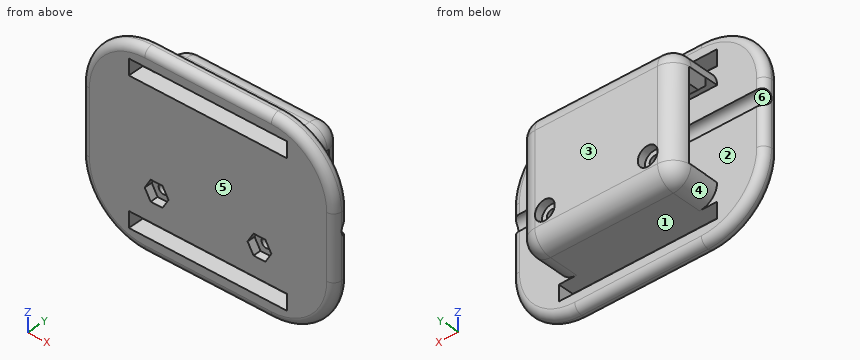
from build123d import *

# Parameters (mm, degrees)
SKETCH1_W               = 31.75
SKETCH1_H               = 25.4
BOSS_EXTRUDE1_DEPTH     = 12.7
SKETCH2_W               = 18.25625
SKETCH2_H               = 6.35
CUT_EXTRUDE3_DEPTH      = 39.058949894
SKETCH4_W               = 1.5875
SKETCH4_H               = 4.7625
BOSS_EXTRUDE2_DEPTH     = 31.75
CUT_EXTRUDE5_DEPTH      = 31.590858593
CUT_EXTRUDE5_DEPTH_BACK = 31.590858593
SKETCH5_R               = 0.9921875
CUT_EXTRUDE6_DEPTH      = 1.5875
SKETCH7_R               = 1.984375
CUT_EXTRUDE7_DEPTH      = 1.5875
SKETCH8_W               = 50.8
SKETCH8_H               = 38.305926372
SKETCH8_W_2             = 31.75
SKETCH8_H_2             = 25.4
BOSS_EXTRUDE3_DEPTH     = 3.175
SKETCH10_W              = 31.75
SKETCH10_H              = 3.175
CUT_EXTRUDE8_DEPTH      = 42.677098196
FILLET6_R               = 12.7
CHAMFER1_SIZE           = 1.016
CHAMFER2_SIZE           = 1.524
FILLET7_R               = 3.556
FILLET10_R              = 1.5875
SKETCH13_R              = 1.5875
CUT_EXTRUDE9_DEPTH      = 74.216005252


# Some blends are built 0.0001 mm under size
with BuildPart() as part:
    # Sketch1 → Boss-Extrude1 (new body)
    with BuildSketch(Plane(origin=(0, 0, 0), x_dir=(1, 0, 0), z_dir=(0, 1, 0))):
        with Locations((7.914574134, 4.007219009)):
            Rectangle(SKETCH1_W, SKETCH1_H)
    extrude(amount=BOSS_EXTRUDE1_DEPTH)

    # Sketch2 → Cut-Extrude3 (cut, through all)
    with BuildSketch(Plane(origin=(23.789574134, 0, 0), x_dir=(0, 0, -1), z_dir=(1, 0, 0))):
        with Locations((4.007219009, 6.35)):
            Rectangle(SKETCH2_W, SKETCH2_H)
    extrude(amount=-CUT_EXTRUDE3_DEPTH, mode=Mode.SUBTRACT)

    # Sketch4 → Boss-Extrude2 (add, through all)
    with BuildSketch(Plane(origin=(23.789574134, 0, 0), x_dir=(0, 0, -1), z_dir=(1, 0, 0))):
        with Locations((-4.327155991, 7.14375)):
            Rectangle(SKETCH4_W, SKETCH4_H)
        with Locations((12.341594009, 7.14375)):
            Rectangle(SKETCH4_W, SKETCH4_H)
    extrude(amount=-BOSS_EXTRUDE2_DEPTH)

    # Sketch5 → Cut-Extrude5 (cut, two sides: drawn at the far end of the back side and taken through both)
    with BuildSketch(Plane(origin=(0, 3.175, 0), x_dir=(1, 0, 0), z_dir=(0, 1, 0)).offset(-CUT_EXTRUDE5_DEPTH_BACK)):
        with Locations(Location((-2.404175866, 10.754094009, 0), (0, 0, 270))):
            Circle(SKETCH5_R)
        with Locations(Location((18.233324134, 10.754094009, 0), (0, 0, 126.869897646))):
            Circle(SKETCH5_R)
    extrude(amount=CUT_EXTRUDE5_DEPTH + CUT_EXTRUDE5_DEPTH_BACK, mode=Mode.SUBTRACT)

    # Sketch6 → Cut-Extrude6 (cut)
    with BuildSketch(Plane.XZ):
        Polygon((-0.022925866, -10.754094009), (-1.213550866, -8.691871016), (-3.594800866, -8.691871016), (-4.785425866, -10.754094009), (-3.594800866, -12.816317002), (-1.213550866, -12.816317002), align=None)
        Polygon((20.614574134, -10.754094009), (19.423949134, -8.691871016), (17.042699134, -8.691871016), (15.852074134, -10.754094009), (17.042699134, -12.816317002), (19.423949134, -12.816317002), align=None)
    extrude(amount=-CUT_EXTRUDE6_DEPTH, mode=Mode.SUBTRACT)

    # Sketch7 → Cut-Extrude7 (cut)
    with BuildSketch(Plane(origin=(0, 12.7, 0), x_dir=(1, 0, 0), z_dir=(0, 1, 0))):
        with Locations(Location((-2.404175866, 10.754094009, 0), (0, 0, 270))):
            Circle(SKETCH7_R)
        with Locations(Location((18.233324134, 10.754094009, 0), (0, 0, 270))):
            Circle(SKETCH7_R)
    extrude(amount=-CUT_EXTRUDE7_DEPTH, mode=Mode.SUBTRACT)

    # Sketch8 → Boss-Extrude3 (add)
    with BuildSketch(Plane.XZ):
        with Locations((7.914574134, -4.007219009)):
            Rectangle(SKETCH8_W, SKETCH8_H)
        with Locations((7.914574134, -4.007219009)):
            Rectangle(SKETCH8_W_2, SKETCH8_H_2, mode=Mode.SUBTRACT)
    extrude(amount=-BOSS_EXTRUDE3_DEPTH)

    # Sketch10 → Cut-Extrude8 (cut, through all)
    with BuildSketch(Plane(origin=(0, 3.175, 0), x_dir=(1, 0, 0), z_dir=(0, 1, 0))):
        with Locations((7.914574134, 18.294719009)):
            Rectangle(SKETCH10_W, SKETCH10_H)
        with Locations((7.914574134, -10.280280991)):
            Rectangle(SKETCH10_W, SKETCH10_H)
    extrude(amount=-CUT_EXTRUDE8_DEPTH, mode=Mode.SUBTRACT)

    # Fillet6
    fillet6_edges = [part.edges().sort_by_distance(p)[0] for p in [
        (-17.485425866, 1.5875, 15.145744177),
        (33.314574134, 1.5875, 15.145744177),
        (33.314574134, 1.5875, -23.160182195),
        (-17.485425866, 1.5875, -23.160182195),
    ]]
    fillet(fillet6_edges, radius=FILLET6_R)

    # Chamfer1
    # the kernel refuses this chamfer: 1.016 mm, written as the material it takes off along each edge
    with BuildSketch(Plane(origin=(-7.960425866, 4.7625, 0.920576075), x_dir=(-0.027495876610586435, 0.9996219169112968, 0), z_dir=(0, 0, 1)), Plane(origin=(-7.960425866, 4.7625, -13.135344009), x_dir=(-0.027495876610586435, 0.9996219169112968, 1.1185418764848949e-15), z_dir=(0, 0, 1))) as chamfer1_piece_1:
        Polygon((CHAMFER1_SIZE * 0.999621916911, -CHAMFER1_SIZE * 0.0274958766106), (-CHAMFER1_SIZE * 0.0274958766106, -CHAMFER1_SIZE * 0.999621916911), (0, 0), align=None)
    extrude(amount=4.200329916, mode=Mode.SUBTRACT)
    with BuildSketch(Plane(origin=(26.402404049, 4.7625, 3.533405991), x_dir=(0, 0.9996219169112968, -0.027495876610586435), z_dir=(-1, 0, 0))) as chamfer1_piece_2:
        Polygon((CHAMFER1_SIZE * 0.999621916911, -CHAMFER1_SIZE * 0.0274958766106), (-CHAMFER1_SIZE * 0.0274958766106, -CHAMFER1_SIZE * 0.999621916911), (0, 0), align=None)
    extrude(amount=36.975659832, mode=Mode.SUBTRACT)
    with BuildSketch(Plane(origin=(23.789574134, 4.7625, 0.920576075), x_dir=(0.027495876610587285, 0.9996219169112968, 0), z_dir=(0, 0, 1)), Plane(origin=(23.789574134, 4.7625, -13.135344009), x_dir=(0.027495876610587285, 0.9996219169112968, 1.1185418764848949e-15), z_dir=(0, 0, 1))) as chamfer1_piece_3:
        Polygon((CHAMFER1_SIZE * 0.999621916911, CHAMFER1_SIZE * 0.0274958766106), (-CHAMFER1_SIZE * 0.0274958766106, CHAMFER1_SIZE * 0.999621916911), (0, 0), align=None)
    extrude(amount=4.200329916, mode=Mode.SUBTRACT)
    with BuildSketch(Plane(origin=(-0.386658451, 4.7625, -11.547844009), x_dir=(0, -0.027495876610585605, -0.9996219169112968), z_dir=(-1, 0, 0)), Plane(origin=(26.402404049, 4.7625, -11.547844009), x_dir=(0, -0.027495876610585605, -0.9996219169112968), z_dir=(-1, 0, 0))) as chamfer1_piece_4:
        Polygon((CHAMFER1_SIZE * 0.999621916911, -CHAMFER1_SIZE * 0.0274958766106), (-CHAMFER1_SIZE * 0.0274958766106, -CHAMFER1_SIZE * 0.999621916911), (0, 0), align=None)
    extrude(amount=10.186597332, mode=Mode.SUBTRACT)
    with BuildSketch(Plane(origin=(20.250841549, 4.7625, -11.547844009), x_dir=(0, -0.027495876610585605, -0.9996219169112968), z_dir=(-1, 0, 0))) as chamfer1_piece_5:
        Polygon((CHAMFER1_SIZE * 0.999621916911, -CHAMFER1_SIZE * 0.0274958766106), (-CHAMFER1_SIZE * 0.0274958766106, -CHAMFER1_SIZE * 0.999621916911), (0, 0), align=None)
    extrude(amount=24.672534832, mode=Mode.SUBTRACT)

    # Chamfer2
    chamfer2_edges = [part.edges().sort_by_distance(p)[0] for p in [
        (-7.960425866, 7.65175, 3.533405991),
        (23.789574134, 7.65175, 3.533405991),
        (-7.960425866, 7.65175, -11.547844009),
        (23.789574134, 7.65175, -11.547844009),
    ]]
    chamfer(chamfer2_edges, length=CHAMFER2_SIZE)

    # Fillet7
    # the kernel refuses this fillet: 3.556 mm, written as the material it takes off along each edge
    with BuildSketch(Plane(origin=(20.233574134, 9.144, 5.136780991), x_dir=(0, 0, 1), z_dir=(1, 0, 0))) as fillet7_piece_1_section:
        Polygon((0, 0), (FILLET7_R * 1.02, 0), (FILLET7_R * 1.02, -FILLET7_R * 1.02), (0, -FILLET7_R * 1.02), align=None)
    fillet7_piece_1 = extrude(amount=FILLET7_R * 1.02, mode=Mode.PRIVATE)
    fillet7_piece_1 = fillet7_piece_1 - Plane(origin=(20.233574134, 9.144, 5.136780991), x_dir=(0, -0.7071067811865475, -0.7071067811865475), z_dir=(1, 0, 0)) * Sphere(FILLET7_R, mode=Mode.PRIVATE)
    add(fillet7_piece_1, mode=Mode.SUBTRACT)
    with BuildSketch(Plane(origin=(-4.404425866, 9.144, 5.136780991), x_dir=(0, 0, 1), z_dir=(-1, 0, 0))) as fillet7_piece_2_section:
        Polygon((0, 0), (FILLET7_R * 1.02, 0), (FILLET7_R * 1.02, FILLET7_R * 1.02), (0, FILLET7_R * 1.02), align=None)
    fillet7_piece_2 = extrude(amount=FILLET7_R * 1.02, mode=Mode.PRIVATE)
    fillet7_piece_2 = fillet7_piece_2 - Plane(origin=(-4.404425866, 9.144, 5.136780991), x_dir=(0, -0.7071067811865475, -0.7071067811865475), z_dir=(-1, 0, 0)) * Sphere(FILLET7_R, mode=Mode.PRIVATE)
    add(fillet7_piece_2, mode=Mode.SUBTRACT)
    with BuildSketch(Plane(origin=(20.233574134, 9.144, -13.151219009), x_dir=(1, 0, 0), z_dir=(0, 0, -1))) as fillet7_piece_3_section:
        Polygon((0, 0), (FILLET7_R * 1.02, 0), (FILLET7_R * 1.02, -FILLET7_R * 1.02), (0, -FILLET7_R * 1.02), align=None)
    fillet7_piece_3 = extrude(amount=FILLET7_R * 1.02, mode=Mode.PRIVATE)
    fillet7_piece_3 = fillet7_piece_3 - Plane(origin=(20.233574134, 9.144, -13.151219009), x_dir=(-0.7071067811865475, -0.7071067811865475, 0), z_dir=(0, 0, -1)) * Sphere(FILLET7_R, mode=Mode.PRIVATE)
    add(fillet7_piece_3, mode=Mode.SUBTRACT)
    with BuildSketch(Plane(origin=(-4.404425866, 9.144, -13.151219009), x_dir=(-1, 0, 0), z_dir=(0, 0, -1))) as fillet7_piece_4_section:
        Polygon((0, 0), (FILLET7_R * 1.02, 0), (FILLET7_R * 1.02, FILLET7_R * 1.02), (0, FILLET7_R * 1.02), align=None)
    fillet7_piece_4 = extrude(amount=FILLET7_R * 1.02, mode=Mode.PRIVATE)
    fillet7_piece_4 = fillet7_piece_4 - Plane(origin=(-4.404425866, 9.144, -13.151219009), x_dir=(0.7071067811865475, -0.7071067811865475, 0), z_dir=(0, 0, -1)) * Sphere(FILLET7_R, mode=Mode.PRIVATE)
    add(fillet7_piece_4, mode=Mode.SUBTRACT)
    with BuildSketch(Plane(origin=(20.233574134, 12.7, 8.692780991), x_dir=(0, -1, 0), z_dir=(-1, 0, 0))) as fillet7_piece_5:
        with BuildLine():
            CenterArc((FILLET7_R, -FILLET7_R), FILLET7_R, 90, 90)
            Line((0, -FILLET7_R), (0, 0))
            Line((0, 0), (FILLET7_R, 0))
        make_face()
    extrude(amount=24.638, mode=Mode.SUBTRACT)
    with BuildSketch(Plane(origin=(23.789574134, 3.175, 8.692780991), x_dir=(-1, 0, 0), z_dir=(0, 1, 0)), Plane(origin=(-7.960425866, 3.175, -16.707219009), x_dir=(1, 0, 0), z_dir=(0, 1, 0))) as fillet7_piece_6:
        with BuildLine():
            CenterArc((FILLET7_R, -FILLET7_R), FILLET7_R, 90, 90)
            Line((0, -FILLET7_R), (0, 0))
            Line((0, 0), (FILLET7_R, 0))
        make_face()
    extrude(amount=5.969, mode=Mode.SUBTRACT)
    with BuildSketch(Plane(origin=(23.789574134, 12.7, -13.151219009), x_dir=(-1, 0, 0), z_dir=(0, 0, 1)), Plane(origin=(-7.960425866, 12.7, 5.136780991), x_dir=(1, 0, 0), z_dir=(0, 0, -1))) as fillet7_piece_7:
        with BuildLine():
            CenterArc((FILLET7_R, FILLET7_R), FILLET7_R, 180, 90)
            Line((0, FILLET7_R), (0, 0))
            Line((0, 0), (FILLET7_R, 0))
        make_face()
    extrude(amount=18.288, mode=Mode.SUBTRACT)
    with BuildSketch(Plane(origin=(23.789574134, 3.175, -16.707219009), x_dir=(-1, 0, 0), z_dir=(0, 1, 0)), Plane(origin=(-7.960425866, 3.175, 8.692780991), x_dir=(1, 0, 0), z_dir=(0, 1, 0))) as fillet7_piece_8:
        with BuildLine():
            CenterArc((FILLET7_R, FILLET7_R), FILLET7_R, 180, 90)
            Line((0, FILLET7_R), (0, 0))
            Line((0, 0), (FILLET7_R, 0))
        make_face()
    extrude(amount=5.969, mode=Mode.SUBTRACT)
    with BuildSketch(Plane(origin=(-4.404425866, 12.7, -16.707219009), x_dir=(0, 0, 1), z_dir=(1, 0, 0))) as fillet7_piece_9:
        with BuildLine():
            CenterArc((FILLET7_R, FILLET7_R), FILLET7_R, 180, 90)
            Line((0, FILLET7_R), (0, 0))
            Line((0, 0), (FILLET7_R, 0))
        make_face()
    extrude(amount=24.638, mode=Mode.SUBTRACT)

    # Fillet10
    fillet10_edges = [part.edges().sort_by_distance(p)[0] for p in [
        (7.914574134, 3.175, 15.145744177),
        (7.914574134, 0, 15.145744177),
        (-17.485425866, 0, -4.007219009),
        (7.914574134, 0, -23.160182195),
        (33.314574134, 0, -4.007219009),
        (29.594830255, 0, 11.426000298),
        (29.594830255, 0, -19.440438316),
        (-13.765681988, 0, -19.440438316),
        (-13.765681988, 0, 11.426000298),
        (-17.485425866, 3.175, -4.007219009),
        (33.314574134, 3.175, -4.007219009),
        (7.914574134, 3.175, -23.160182195),
    ]]
    fillet(fillet10_edges, radius=FILLET10_R - 0.0001)  # a hair under: the kernel refuses the full size

    # Sketch13 → Cut-Extrude9 (cut, through all)
    with BuildSketch(Plane(origin=(50.8, 0, 0), x_dir=(0, 0, -1), z_dir=(1, 0, 0))):
        with Locations((1.213219009, 3.175)):
            Circle(SKETCH13_R)
    extrude(amount=-CUT_EXTRUDE9_DEPTH, mode=Mode.SUBTRACT)


solid = part.part
Could you check a few things on this model? Use its own coordinates, in mm. Face numbers are marked on the shaded views. A direction names the side the tool comes from. Coordinates: 2 decimals unless noted, no trailing zeros. Order: outer loops, then holes, each group sorted by start corner. A loop starts at its lowest first (then second) coordinate and runs counter-clockwise, first axis right, second up. Notation, with made-up numbers: (61.5, 21.25) -> (96.5, 21.25) arc R15 cw to (96.5, 38.25) -> close; hole circle Ø9 at (-39, 7.25). An arc over 180 degrees is marked (long way). One line per item, written item: value. Start each with the question number.
1) Imagine slicing it at B-B on y = 6.75. List the corners of the cut face in (x, z) for me, plus the area to 3 significant figures.
2) I'm going to push flat-ended pins straight in: pin 1 (4 mm diameter, centred on x = 6, y = 7.5, fed in from +Z); pin 2 (2.5 mm diameter, centred on x = 18.23, z = -10.75, fed in from +Y); pin 3 (3.5 mm diameter, centred on y = 1.5, z = 10.5, fed in from -X); pin 4 (1.2 mm diameter, centred on x = -2.4, z = -10.75, fed in from -Y). Where does each tip first touch, or does it pass through?
3) We'd pull the mould along Z, two halves only. Please class the marked faces 1, 2, 3 and 4: +Z half, -Z half, draft (parallel to the pull), parting line (faces both ways), or undercut.
4) Which directions (+Z, -Z, +X, -X, +Y, -Y) give clear straight access to the entire face, cutting with the end or side of a thin tool? Please do the marked faces 5 and 6.
5) If I drill on L1, parallel to Y at x = 11, z = 5 (1 decimal); L2, parallel to Z at x = 12, y = 2; L3, parallel to Y at x = 0, z = 13 (3 decimals), over which ranges is the centre line in solid material (lowest first)? Write a range as [from, to].
6) Imagine slicing it at D-D on y = 10.5. List the corners of the cut face in (x, z) for me.
7) Imagine slicing it at A-A on x = 11. Count the separate pieces of the cut face and the enclosed holes in it, plus the area to 3 significant figures.
Answer list:
1. outline: (-7.96, -13.15) arc R3.56 ccw to (-4.4, -16.71) -> (20.23, -16.71) arc R3.56 ccw to (23.79, -13.15) -> (23.79, -13.07) -> (22.27, -11.55) -> (18.83, -11.55) arc R0.99 cw to (17.64, -11.55) -> (-1.81, -11.55) arc R0.99 cw to (-3, -11.55) -> (-6.44, -11.55) -> (-7.96, -13.07) -> close; (-7.96, 5.06) -> (-6.44, 3.53) -> (22.27, 3.53) -> (23.79, 5.06) -> (23.79, 5.14) arc R3.56 ccw to (20.23, 8.69) -> (-4.4, 8.69) arc R3.56 ccw to (-7.96, 5.14) -> close
1. area: 312 mm2
2. pin 1: stops at z = 8.69
2. pin 2: stops at y = 11.11
2. pin 3: stops at x = -15.81
2. pin 4: passes through
3. face 1: undercut
3. face 2: undercut
3. face 3: draft
3. face 4: -Z half
4. face 5: +Z, -Z, +X, -X, -Y
4. face 6: +X, -X
5. L1: y = [0, 3.2], [4.8, 12.7]
5. L2: z = [-23.11, -19.88], [-16.71, -2.28], [-0.15, 8.69], [11.87, 15.09]
5. L3: y = [0, 3.175]
6. outline: (-7.69, -13.15) arc R3.29 ccw to (-4.4, -16.44) -> (20.23, -16.44) arc R3.29 ccw to (23.52, -13.15) -> (23.52, 5.14) arc R3.29 ccw to (20.23, 8.42) -> (-4.4, 8.42) arc R3.29 ccw to (-7.69, 5.14) -> close; hole circle Ø1.98 at (-2.4, -10.75); hole circle Ø1.98 at (18.23, -10.75)
7. separate pieces: 3
7. enclosed holes: 1
7. area: 230 mm2
